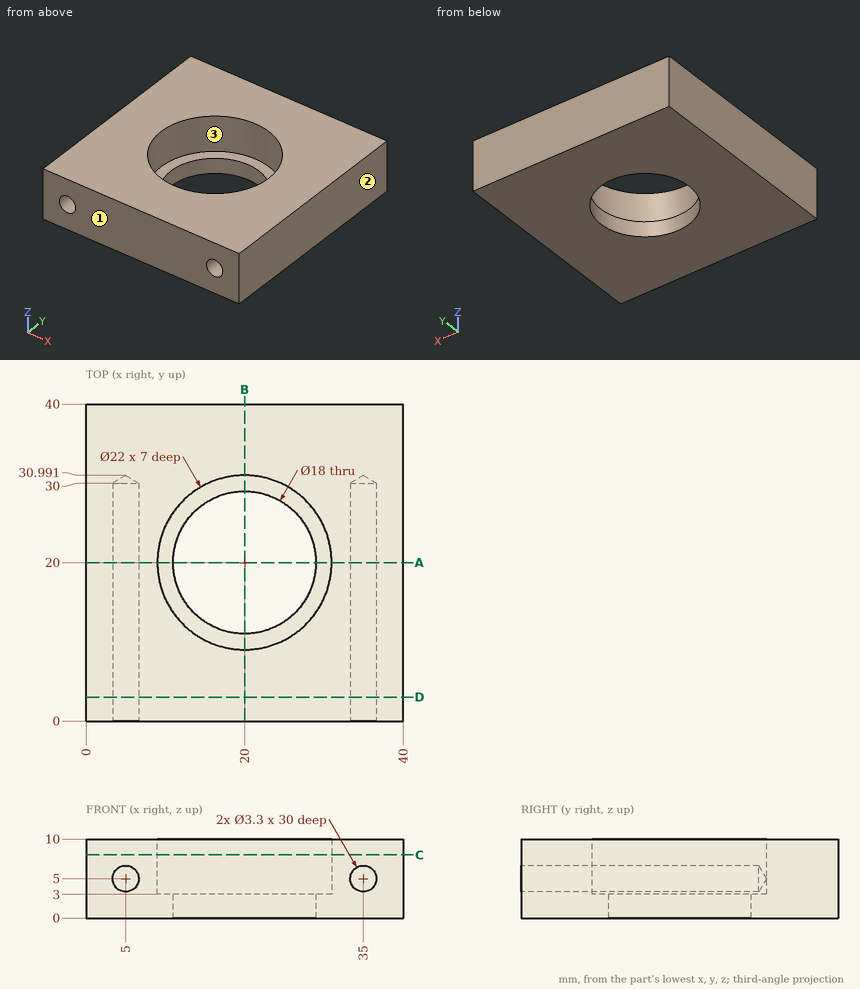
Check sheet for the drawn part. Datum: minimum x, y, z corner. Units: mm. Give positions to 0.01 mm unless a question says otherwise; leave off trailing zeros. Order: outer loops, then holes, each group sorted by start corner. A loop starts at its lowest first (then second) coordinate and runs counter-clockwise, first axis right, second up. Notation, with made-up numbers: (49, -3.75) - (68, -3.75) arc R14 cw to (68, 8.25) - close; hole circle Ø1 at (-32, 7.5). An arc over 180 degrees is marked (long way). Write item = value, one per line. Start each with the question number.
1) Scan lines: L1, parallel to X at y = 29, z = 6.5 (1 decimal); L2, parallel to X at y = 14.5, z = 3.75 (1 decimal); L3, parallel to Y at x = 20, z = 0.7. Record each from-to range of solid material in increasing order.
2) Section check D-D (y = 3). Enter the section's corners in (x, z).
3) Section check B-B (x = 20). Enter the section's corners in (y, z).
4) Gauge pin test, flat ends, axial feed: pin 1 Ø3 at (x, z) = (5, 5) entering from -Y; pin 2 Ø3 at (x, y) = (19.5, 11.5) entering from +Z. Record the tip position at first contact, or that the pin passes through.
5) Section check C-C (z = 8). Enter the section's corners in (x, y).
6) Section check A-A (y = 20). Enter the section's corners in (x, z).
7) Draft check along X on the marked faces 1, 2 and 3. Enter one of: released by +X, released by -X, zero draft, split by the parting line, or undercut.
Geometry check:
q1.L1 = 0 to 4.3, 5.7 to 13.7, 26.3 to 34.3, 35.7 to 40
q1.L2 = 0 to 3.9, 6.1 to 10.5, 29.5 to 33.9, 36.1 to 40
q1.L3 = 0 to 11, 29 to 40
q2.outline = (0, 0) - (40, 0) - (40, 10) - (0, 10) - close; hole circle Ø3.3 at (5, 5); hole circle Ø3.3 at (35, 5)
q3.outline = (0, 0) - (11, 0) - (11, 3) - (9, 3) - (9, 10) - (0, 10) - close; (29, 0) - (40, 0) - (40, 10) - (31, 10) - (31, 3) - (29, 3) - close
q4.pin_1 = 30.09
q4.pin_2 = 3
q5.outline = (0, 0) - (40, 0) - (40, 40) - (0, 40) - close; hole circle Ø22 at (20, 20)
q6.outline = (0, 0) - (11, 0) - (11, 3) - (9, 3) - (9, 10) - (0, 10) - close; (29, 0) - (40, 0) - (40, 10) - (31, 10) - (31, 3) - (29, 3) - close; hole circle Ø3.3 at (5, 5); hole circle Ø3.3 at (35, 5)
q7.face_1 = zero draft
q7.face_2 = released by +X
q7.face_3 = undercut
